Source: CAD feature listing. Evaluate the final solid. Frame: model axes, mm. A direction names the side the tool comes from. Give positions to 0.01 mm unless a question says otherwise; leave off trailing zeros. Write each loop counter-clockwise with the first axis right and the second up, starting at its lowest first coordinate (ties: lowest second). Pieces come first, ordered by that corner, then holes. Notation, with made-up numbers: (-10, 53.25) - (20, 53.25) arc R24 cw to (20, 86.25) - close; hole circle Ø4 at (17.5, 76.5). An arc over 180 degrees is marked (long way). One line per question, with ' | ' between items. Start each with the question number.
(1) Draft query along Z for faces 3 (the flat face through (10, -198, -223)), 4 (the cylindrical face through (1.479, -186.458, -370.273)), 5 (the cylindrical face through (4.93, -315.26, -8.555)). Return one class per face: +Z half, -Z half, draft (parallel to the pull), parting line (faces both ways), or undercut.
(2) Access query for faces 1 (the flat face through (3, -161, -212)), 2 (the cylindrical face through (4.93, -6.014, -4.375)). Directions: +Z, -Z, +X, -X, +Y, -Y. A direction counts if a zero-diameter tool reaches every point of the face in a straight line with its end or side. Return the directions, or none.
(3) Pin query (flat end, axial travel): pin 1 (4 mm diameter, centred on x = 5, z = -291, fed in from +Y); pin 2 (3 mm diameter, centred on x = 8.5, z = -284.5, fed in from +Y); pin 3 (6 mm diameter, centred on y = -150, z = -130.5, fed in from -X). Return the tip coordinate at first contact, or that it passes through.
(4) Ray query, line 1 (X direction, y = -232, z = -118.5); line 2 (Y direction, x = 8, z = -131); line 3 (Y direction, x = 1.5, z = -477.5). Return the intervals inside material, ascending. Write a range as [from, to].
(5) Section A-A, the plane x = 8.25. Return loops of the section in (y, z), plus the area to 3 significant figures.
```python
from build123d import *

# Parameters (mm, degrees)
BOSS_EXTRUDE1_DEPTH = 10
CUT_EXTRUDE3_DEPTH  = 3


with BuildPart() as part:
    # Sketch1 → Boss-Extrude1 (new body)
    with BuildSketch(Plane(origin=(0, 0, 0), x_dir=(0, 0, -1), z_dir=(1, 0, 0))):
        with BuildLine():
            Line((0, -14.281480067), (0, -294.281480067))
            ThreePointArc((0, -294.281480067), (8.786796564, -315.494683503), (30, -324.281480067))
            Line((30, -324.281480067), (573.815572472, -324.281480067))
            ThreePointArc((573.815572472, -324.281480067), (580.886640283, -321.352547879), (583.815572472, -314.281480067))
            Line((583.815572472, -314.281480067), (583.815572472, -219.493566063))
            ThreePointArc((583.815572472, -219.493566063), (582.007092914, -213.757801699), (577.235773905, -210.096639855))
            Line((577.235773905, -210.096639855), (13.420201433, -4.88455386))
            ThreePointArc((13.420201433, -4.88455386), (4.264235636, -6.089959625), (0, -14.281480067))
        make_face()
    extrude(amount=BOSS_EXTRUDE1_DEPTH)

    # Sketch3 → Cut-Extrude3 (cut)
    with BuildSketch(Plane.ZY):
        with BuildLine():
            ThreePointArc((-23.162175785, -218.017297737), (-17.576945532, -207.678107035), (-26.738120061, -200.318314743))
            add(Edge.make_bspline(
                [(-26.738120061, -200.318314743), (-45.914354434, -200.660753587), (-151.32107334, -255.510398156), (-414.880335601, -286.385074175), (-542.431128002, -257.731725159), (-546.154906269, -257.731029979)],
                knots=[0, 0, 0, 0, 0.560935224, 0.660935224, 1, 1, 1, 1], degree=3))
            ThreePointArc((-546.154906269, -257.731029979), (-563.288388976, -273.27487263), (-549.474047026, -291.831036849))
            add(Edge.make_bspline(
                [(-549.474047026, -291.831036849), (-474.750080899, -306.502271197), (-284.669923623, -324.572171749), (-143.080818041, -266.034178467), (-23.162175785, -218.017297737)],
                knots=[0, 0, 0, 0, 0.423888314, 1, 1, 1, 1], degree=3))
        make_face()
        with BuildLine():
            ThreePointArc((-26.950185671, -47.737214996), (-28.17113687, -40.715672082), (-35.124917897, -39.154353359))
            add(Edge.make_bspline(
                [(-35.124917897, -39.154353359), (-50.602952828, -45.122445935), (-99.042539, -170.661871263), (-331.224003862, -171.181746235), (-353.169530365, -171.181734297)],
                knots=[0, 0, 0, 0, 0.639195597, 1, 1, 1, 1], degree=3))
            ThreePointArc((-353.169530365, -171.181734297), (-370.309371751, -186.812434708), (-356.32010769, -205.316311305))
            add(Edge.make_bspline(
                [(-356.32010769, -205.316311305), (-352.838937223, -205.964445921), (-121.396454164, -217.989087479), (-35.312726243, -66.629555086), (-26.950185671, -47.737214996)],
                knots=[0, 0, 0, 0, 0.40968467, 1, 1, 1, 1], degree=3))
        make_face()
    extrude(amount=-CUT_EXTRUDE3_DEPTH, mode=Mode.SUBTRACT)


solid = part.part
```
Check sheet entries:
1) face 3: draft | face 4: undercut | face 5: +Z half
2) face 1: -X | face 2: +X, -X, +Y
3) pin 1: y = -105.19 | pin 2: y = -103 | pin 3: x = 3
4) line 1: [3, 10] | line 2: [-324.28, -47.68] | line 3: [-324.28, -303.41], [-269.07, -173.8]
5) outline: (-324.28, -573.82) arc R10 ccw to (-314.28, -583.82) - (-219.49, -583.82) arc R10 ccw to (-210.1, -577.24) - (-4.88, -13.42) arc R10 ccw to (-14.28, 0) - (-294.28, 0) arc R30 ccw to (-324.28, -30) - close | area: 127,000 mm²
